Can you work these out from the drawing? Everything is in mm from the part's minimum corner. Give positions to 0.01 mm unless a question says otherwise; leave off trailing zeros. Order: outer loops, then holes, each group sorted by start corner. A loop starts at its lowest first (then second) coordinate and runs counter-clockwise, first axis right, second up. Notation, with made-up numbers: M 43,33.5 L 63,33.5 A20 cw 63,40.5 Z; hole C 17.5,-3.5 d8. An arc over 180 degrees is marked long. Use a Markdown table: item, result. Add a question column.
Item 1: Suppose I cut it at C-C on x = 19. Write out the boundary of the cut face in (y, z), plus the area to 3 significant figures.
Item 2: If I drill on L1, parallel to X at y = 143, z = 113; L2, parallel to Y at x = 41.5, z = 80; L3, parallel to Y at x = 31, z = 56, over which ranges is the centre line in solid material (lowest first)? Write a range as from..to.
Item 3: Suppose I cut it at A-A on y = 80. Write out the boundary of the cut face in (x, z).
Item 4: Suppose I cut it at D-D on z = 12. Write out the boundary of the cut face in (x, y).
Item 5: If we mould it in two halves opening along X, with no side actions, what happens to the marked faces 1, 2 and 3? For each: released by +X, released by -X, zero draft, split by the parting line, or undercut.
Item 6: I'm going to push flat-ended pins straight in: pin 1 Ø8 at (x, y) = (19.5, 75) entering from +Z; pin 2 Ø6 at (x, y) = (67.5, 87) entering from -Z; pin 3 Ø1.5 at (x, y) = (45, 64) entering from -Z. Where does each tip first touch, or does it pass through?
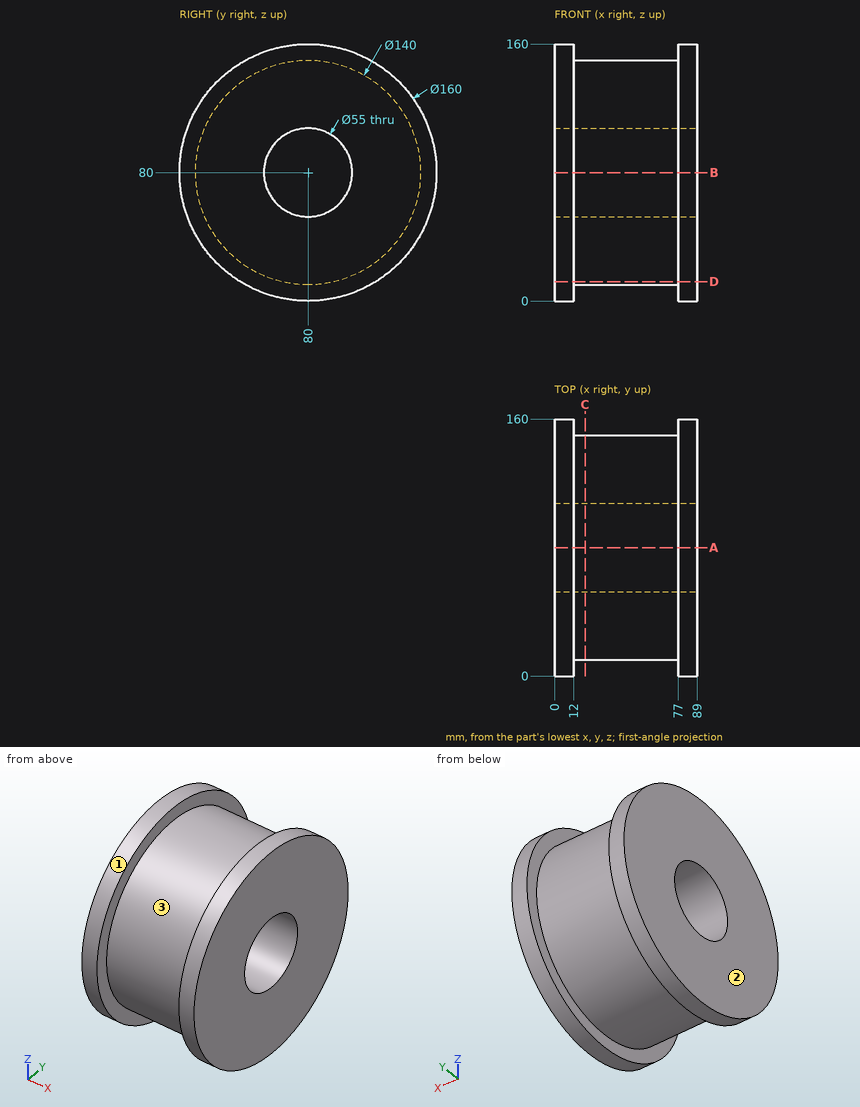
Findings below:
| question | item | result |
|---|---|---|
| 1 | outline | C 80,80 d140; hole C 80,80 d55 |
| 1 | area | 13,000 mm^2 |
| 2 | L1 | x = 0..12, 77..89 |
| 2 | L2 | y = 10..52.5, 107.5..150 |
| 2 | L3 | y = 14.24..66.57, 93.43..145.76 |
| 3 | outline | M 0,0 L 12,0 L 12,10 L 77,10 L 77,0 L 89,0 L 89,52.5 L 0,52.5 Z; M 0,107.5 L 89,107.5 L 89,160 L 77,160 L 77,150 L 12,150 L 12,160 L 0,160 Z |
| 4 | outline | M 0,37.86 L 12,37.86 L 12,63.39 L 77,63.39 L 77,37.86 L 89,37.86 L 89,122.14 L 77,122.14 L 77,96.61 L 12,96.61 L 12,122.14 L 0,122.14 Z |
| 5 | face 1 | zero draft |
| 5 | face 2 | released by -X |
| 5 | face 3 | undercut |
| 6 | pin 1 | stops at z = 149.99 |
| 6 | pin 2 | stops at z = 10.11 |
| 6 | pin 3 | stops at z = 11.68 |
